```python
from build123d import *

# Parameters (mm, degrees)
SKETCH1_W           = 1100
SKETCH1_H           = 22.5
BOSS_EXTRUDE1_DEPTH = 2.5
SKETCH2_W           = 1100
SKETCH2_H           = 2.5
BOSS_EXTRUDE2_DEPTH = 20
SKETCH3_W           = 150
SKETCH3_H           = 20
CUT_EXTRUDE1_DEPTH  = 10
CUT_EXTRUDE2_DEPTH  = 551.57498354
FILLET1_R           = 1


with BuildPart() as part:
    # Sketch1 → Boss-Extrude1 (new body)
    with BuildSketch(Plane(origin=(0, 0, 0), x_dir=(1, 0, 0), z_dir=(0, 1, 0))):
        Rectangle(SKETCH1_W, SKETCH1_H)
    extrude(amount=BOSS_EXTRUDE1_DEPTH)

    # Sketch2 → Boss-Extrude2 (add)
    with BuildSketch(Plane(origin=(0, 2.5, 0), x_dir=(1, 0, 0), z_dir=(0, 1, 0))):
        with Locations((0, 10)):
            Rectangle(SKETCH2_W, SKETCH2_H)
    extrude(amount=BOSS_EXTRUDE2_DEPTH)

    # Sketch3 → Cut-Extrude1 (cut)
    with BuildSketch(Plane.XY.offset(-8.75)):
        with Locations((0, 12.5)):
            Rectangle(SKETCH3_W, SKETCH3_H)
    extrude(amount=-CUT_EXTRUDE1_DEPTH, mode=Mode.SUBTRACT)

    # Sketch4 → Cut-Extrude2 (cut, through all)
    with BuildSketch(Plane(origin=(0, 0, 0), x_dir=(-1, 0, 0), z_dir=(0, -1, 0))):
        Polygon((-550, 11.25), (-527.5, -11.25), (-550, -11.25), align=None)
        Polygon((550, -11.25), (550, 11.25), (527.5, -11.25), align=None)
    extrude(amount=-CUT_EXTRUDE2_DEPTH, mode=Mode.SUBTRACT)

    # Fillet1
    fillet1_edges = [part.edges().sort_by_distance(p)[0] for p in [
        (312.5, 22.5, -11.25),
        (311.25, 22.5, -8.75),
        (-312.5, 22.5, -11.25),
        (311.25, 2.5, -8.75),
        (0, 0, -11.25),
        (0, 0, 11.25),
        (0, 2.5, 11.25),
        (-311.25, 22.5, -8.75),
    ]]
    fillet(fillet1_edges, radius=FILLET1_R)


solid = part.part
```
Work out the finished part from the listing and answer in its coordinate system (mm). A direction names the side the tool comes from. Coordinates: 2 decimals unless noted, no trailing zeros. Loops run counter-clockwise (first coordinate to the right, second up) from the corner with the lowest first, then second, coordinate; pieces in that order, holes last. Notation, with made-up numbers: (48.5, 24.25) - (70.5, 24.25) arc R27 cw to (70.5, 41.25) - close; hole circle Ø9 at (-24, 44.25). An arc over 180 degrees is marked (long way). Use a Markdown table: item, result.
Item 1: Find section D-D, the plane x = -465.5. Determine the outline of the cut face in (y, z), and give its area (3 significant figures).
Evaluation:
| item | result |
|---|---|
| outline | (0, -10.25) arc R1 ccw to (1, -11.25) - (21.5, -11.25) arc R1 ccw to (22.5, -10.25) - (22.5, -9.75) arc R1 ccw to (21.5, -8.75) - (2.5, -8.75) - (2.5, 10.25) arc R1 ccw to (1.5, 11.25) - (1, 11.25) arc R1 ccw to (0, 10.25) - close |
| area | 105 mm2 |
Item 2: For faces 1 (the flat face through (308, 12, -8.75)), 2 (the flat face through (-543.8, 2.03, -5.05)), determine the directions among +Z, -Z, +X, -X, +Y, -Y from which every point of the face is accessible in a straight line to the end or side of a thin tool.
Evaluation:
| item | result |
|---|---|
| face 1 | +Z, +X, -X, +Y |
| face 2 | +Z, -X, +Y, -Y |
Item 3: Given pin 1 Ø3 at (x, z) = (281, -1) entering from +Y; pin 2 Ø6 at (y, z) = (4.5, -3.5) entering from +X; pin 3 Ø1 at (x, y) = (-391, 9) entering from +Z, each flat-ended and moving along its own axis, determine where each tip first touches the part or whether it passes through.
Evaluation:
| item | result |
|---|---|
| pin 1 | stops at y = 2.5 |
| pin 2 | stops at x = 544.49 |
| pin 3 | stops at z = -8.75 |
Item 4: Find section B-B, the plane x = 425. Determine the outline of the cut face in (y, z), and give its area (3 significant figures).
Evaluation:
| item | result |
|---|---|
| outline | (0, -10.25) arc R1 ccw to (1, -11.25) - (21.5, -11.25) arc R1 ccw to (22.5, -10.25) - (22.5, -9.75) arc R1 ccw to (21.5, -8.75) - (3.5, -8.75) arc R1 cw to (2.5, -7.75) - (2.5, 10.25) arc R1 ccw to (1.5, 11.25) - (1, 11.25) arc R1 ccw to (0, 10.25) - close |
| area | 105 mm2 |
Item 5: Consider probe 1 along Z at (x, y) = (-332, 20.5); probe 2 along Y at (x, z) = (59.5, -8); probe 3 along X at (y, z) = (12.75, -9.5). Determine where each line is inside the solid, lowest interval first. Write a range as from..to.
Evaluation:
| item | result |
|---|---|
| probe 1 | z = -11.25..-8.75 |
| probe 2 | y = 0..2.5 |
| probe 3 | x = -548.25..-75, 75..548.25 |
Item 6: Find section C-C, the plane z = -3. Determine the outline of the cut face in (x, y).
Evaluation:
| item | result |
|---|---|
| outline | (-541.75, 0) - (541.75, 0) - (541.75, 2.5) - (-541.75, 2.5) - close |
Item 7: Find section A-A, the plane y = 13.5. Determine the outline of the cut face in (x, z), and give its area (3 significant figures).
Evaluation:
| item | result |
|---|---|
| outline | (-550, -11.25) - (-75, -11.25) - (-75, -8.75) - (-547.5, -8.75) - close; (75, -11.25) - (550, -11.25) - (547.5, -8.75) - (75, -8.75) - close |
| area | 2,370 mm2 |
